```python
from build123d import *

# Parameters (mm, degrees)
F0_W            = 250
F0_H            = 250
F1_DEPTH        = 15
F5_R            = 5
F6_DEPTH        = 15.001
F6_COPIES_COUNT = 7
F6_COPIES_ANGLE = 270
F8_R            = 7.5
F9_DEPTH        = 15.001


# Not quite as in the source:
# - a pattern or mirror of a feature is missing from the dataset's text; its kind, count and spacing are read off the source's solid


with BuildPart() as f1:
    # F0 (on Top) → F1 (new body)
    with BuildSketch(Plane.XY):
        with Locations((-125, 125)):
            Rectangle(F0_W, F0_H)
    extrude(amount=F1_DEPTH)

    # F5 (on face) → F6 (cut, through all)
    with BuildSketch(Plane.XY.offset(15)):
        with Locations((-212.5, 125)):
            Circle(F5_R)
    f6 = extrude(amount=-F6_DEPTH, mode=Mode.SUBTRACT)

    # F6_copies: F6 ×7 about axis
    f6_copies_axis = Axis((-125, 125, 0), (0, 0, -1))
    for i in range(1, F6_COPIES_COUNT):
        add(f6.rotate(f6_copies_axis, i * F6_COPIES_ANGLE / (F6_COPIES_COUNT - 1)), mode=Mode.SUBTRACT)

    # F8 (on face) → F9 (cut, through all)
    with BuildSketch(Plane.XY.offset(15)):
        with Locations((-186.8718433538, 63.1281566462)):
            Circle(F8_R)
    extrude(amount=-F9_DEPTH, mode=Mode.SUBTRACT)


solid = f1.part
```
Work out the finished part from the listing and answer in its coordinate system (mm). Give positions to 0.01 mm unless a question says otherwise; leave off trailing zeros. Order: outer loops, then holes, each group sorted by start corner. A loop starts at its lowest first (then second) coordinate and runs counter-clockwise, first axis right, second up. Notation, with made-up numbers: (8, 2) - (48, 2) arc R9 cw to (48, 6) - close; hole circle Ø11 at (11, -37). An arc over 180 degrees is marked (long way). One line per item, written item: value. Start each with the question number.
1. Section A-A, the plane y = 37.5 is taken. Write down the section's boundary in (x, z), then the cut area to 3 significant figures.
2. Section D-D, the plane x = -37.5 is taken. Write down the section's boundary in (y, z), then the cut area to 3 significant figures.
3. For a pull along Y with two mould halves and no side action, classify faces 1 (the face through (-127, 0, 7)), 2 (the face through (-192.82, 58.56, 7.6)), 3 (the face through (-67.56, 65.44, 7.6)), 4 (the face through (0, 123, 7)) as released by +Y, released by -Y, zero draft, split by the parting line, or undercut.
4. Section B-B, the plane x = -125 is taken. Write down the section's boundary in (y, z).
5. Consider line 1 (Y direction, x = -61, z = 6.25); line 2 (X direction, y = 127, z = 13.75); line 3 (Y direction, x = -67, z = 13.25). Determine where each line is inside the solid, lowest interval first.
6. Section C-C, the plane y = 125 is taken. Write down the section's boundary in (x, z).
Filled sheet:
1. outline: (-250, 0) - (-130, 0) - (-130, 15) - (-250, 15) - close; (-120, 0) - (0, 0) - (0, 15) - (-120, 15) - close
1. area: 3,600 mm²
2. outline: (0, 0) - (120, 0) - (120, 15) - (0, 15) - close; (130, 0) - (250, 0) - (250, 15) - (130, 15) - close
2. area: 3,600 mm²
3. face 1: released by -Y
3. face 2: undercut
3. face 3: undercut
3. face 4: zero draft
4. outline: (0, 0) - (32.5, 0) - (32.5, 15) - (0, 15) - close; (42.5, 0) - (207.5, 0) - (207.5, 15) - (42.5, 15) - close; (217.5, 0) - (250, 0) - (250, 15) - (217.5, 15) - close
5. line 1: 0 to 58.6, 67.65 to 182.35, 191.4 to 250
5. line 2: -250 to -217.08, -207.92 to -42.08, -32.92 to 0
5. line 3: 0 to 59.96, 66.29 to 183.71, 190.04 to 250
6. outline: (-250, 0) - (-217.5, 0) - (-217.5, 15) - (-250, 15) - close; (-207.5, 0) - (-42.5, 0) - (-42.5, 15) - (-207.5, 15) - close; (-32.5, 0) - (0, 0) - (0, 15) - (-32.5, 15) - close
